Can you work these out from the model? Positions are in its coordinate system, mm. Round coordinates to 2 decimals unless told otherwise and drop trailing zeros. Loops run counter-clockwise (first coordinate to the right, second up) from the corner with the lowest first, then second, coordinate; pieces in that order, holes last.
(1) If I drill on line 1 along Z through (x, y) = (4.5, 1.4); line 2 along X through (y, z) = (0.8, 5), over which ranges is the centre line in solid material (lowest first)?
(2) I want a section at B-B on x = 9. Write out the boundary of the cut face in (y, z), plus the area to 3 significant figures.
(3) I want a section at C-C on y = 0.35. Give the number of separate pieces and of enclosed holes in the cut face, plus the area to 4 significant figures.
(4) I want a section at A-A on z = 7. Write out the boundary of the cut face in (x, y), plus the area to 3 significant figures.
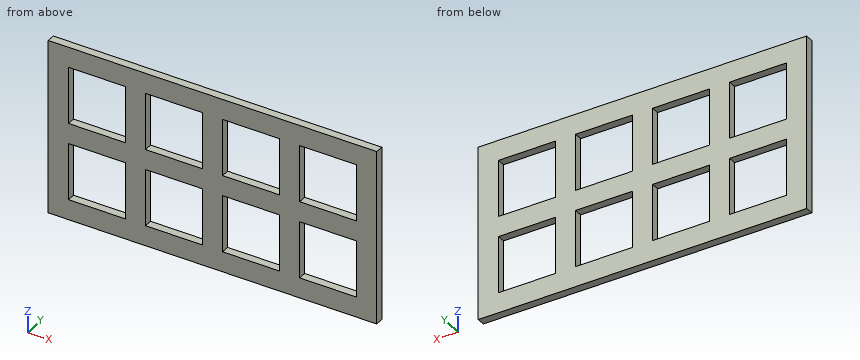
from build123d import *

# Parameters (mm, degrees)
SKETCH1_W           = 14
SKETCH1_H           = 14
BOSS_EXTRUDE1_DEPTH = 2


with BuildPart() as part:
    # Sketch1 → Boss-Extrude1 (new body)
    with BuildSketch(Plane(origin=(0, 0, 0), x_dir=(1, 0, 0), z_dir=(0, 1, 0))):
        Polygon((-40.5, 21.5), (40.5, 21.5), (40.5, 16.5), (40.5, 0), (40.5, -16.5), (40.5, -21.5), (-40.5, -21.5), (-40.5, -16.5), (-40.5, 16.5), align=None)
        with Locations((28.5, 9.5)):
            Rectangle(SKETCH1_W, SKETCH1_H, mode=Mode.SUBTRACT)
        with Locations((9.5, 9.5)):
            Rectangle(SKETCH1_W, SKETCH1_H, mode=Mode.SUBTRACT)
        with Locations((-28.5, 9.5)):
            Rectangle(SKETCH1_W, SKETCH1_H, mode=Mode.SUBTRACT)
        with Locations((-9.5, 9.5)):
            Rectangle(SKETCH1_W, SKETCH1_H, mode=Mode.SUBTRACT)
        with Locations((-28.5, -9.5)):
            Rectangle(SKETCH1_W, SKETCH1_H, mode=Mode.SUBTRACT)
        with Locations((-9.5, -9.5)):
            Rectangle(SKETCH1_W, SKETCH1_H, mode=Mode.SUBTRACT)
        with Locations((28.5, -9.5)):
            Rectangle(SKETCH1_W, SKETCH1_H, mode=Mode.SUBTRACT)
        with Locations((9.5, -9.5)):
            Rectangle(SKETCH1_W, SKETCH1_H, mode=Mode.SUBTRACT)
    extrude(amount=BOSS_EXTRUDE1_DEPTH)


solid = part.part
Filled sheet:
1. line 1: z = -21.5 to -16.5, -2.5 to 2.5, 16.5 to 21.5
1. line 2: x = -40.5 to -35.5, -21.5 to -16.5, -2.5 to 2.5, 16.5 to 21.5, 35.5 to 40.5
2. outline: (0, -21.5) - (2, -21.5) - (2, -16.5) - (0, -16.5) - close; (0, -2.5) - (2, -2.5) - (2, 2.5) - (0, 2.5) - close; (0, 16.5) - (2, 16.5) - (2, 21.5) - (0, 21.5) - close
2. area: 30.0 mm2
3. separate pieces: 1
3. enclosed holes: 8
3. area: 1,915 mm2
4. outline: (-40.5, 0) - (-35.5, 0) - (-35.5, 2) - (-40.5, 2) - close; (-21.5, 0) - (-16.5, 0) - (-16.5, 2) - (-21.5, 2) - close; (-2.5, 0) - (2.5, 0) - (2.5, 2) - (-2.5, 2) - close; (16.5, 0) - (21.5, 0) - (21.5, 2) - (16.5, 2) - close; (35.5, 0) - (40.5, 0) - (40.5, 2) - (35.5, 2) - close
4. area: 50.0 mm2
